CAD build for the part. Positions are in the model's coordinates, mm. A direction names the side the tool comes from. Coordinates: 2 decimals unless noted, no trailing zeros. Loops run counter-clockwise (first coordinate to the right, second up) from the corner with the lowest first, then second, coordinate; pieces in that order, holes last. Notation, with made-up numbers: (-28, 0.5) -> (26, 0.5) arc R6 cw to (26, 8.5) -> close; hole circle Ø3 at (57, -3.5). An arc over 180 degrees is marked (long way). Write each question's results on one line, items separated by ' | '.
Autodesk Inventor part; units mm, degrees
ref_plane "Work Plane1" through (0, -2.54, 0) normal (0, -1, 0) x (1, 0, 0)
ref_plane "YZ Plane" through (0, 0, 0) normal (1, 0, 0) x (0, 1, 0)
ref_plane "XZ Plane" through (0, 0, 0) normal (0, 1, 0) x (-1, 0, 0)
sketch "Sketch1" plane through (0, 0, 0) normal (0, 1, 0) x (-1, 0, 0)
  arc A0 (8.89, 11.1125) -> (-8.89, 11.1125) centre (0, 11.1125) ccw
  line L0 (-8.89, 0) -> (8.89, 0)
  arc A1 (-8.89, -11.1125) -> (8.89, -11.1125) centre (0, -11.1125) ccw
  line L1 (8.89, 11.1125) -> (8.89, -11.1125)
  line L2 (-8.89, 11.1125) -> (-8.89, -11.1125)
  point P0 (0, 0)
extrude "Extrusion1" add sketch "Sketch1" along normal blind 5.588
sketch "Sketch2" plane through (0, 5.588, 0) normal (0, 1, 0) x (1, 0, 0)
  arc A0 (-7.62, -11.1125) -> (7.62, -11.1125) centre (0, -11.1125) ccw
  arc A1 (7.62, 11.1125) -> (-7.62, 11.1125) centre (0, 11.1125) ccw
  line L0 (-7.62, -11.1125) -> (-7.62, 11.1125)
  line L1 (7.62, -11.1125) -> (7.62, 11.1125)
  line L2 (8.89, -11.1125) -> (8.89, 11.1125)
  line L3 (-8.89, 11.1125) -> (-8.89, -11.1125)
  arc A2 (-8.89, -11.1125) -> (8.89, -11.1125) centre (0, -11.1125) ccw
  point P0 (0, 0)
  dimension "d32" = 1.27
  dimension "d33" = 1.27
  dimension "d34" = 1.27
  dimension "d36" = 22.225
  dimension "d37" = 22.225
  dimension "d38" = 22.225
extrude "Extrusion2" cut sketch "Sketch2" against normal blind 0.508
sketch "Sketch3" plane through (0, 5.08, 0) normal (0, 1, 0) x (1, 0, 0)
  circle A0 centre (0, 0) radius 3.175
  point P0 (0, 0)
  dimension "d10" = 6.35
hole "Hole1" at (0, 5.08, 0) direction (0, -1, 0) diameter 6.35 end through all
thread "Thread1"
sketch "Sketch4" plane through (8.89, 0, 11.1125) normal (1, 0, 0) x (0, 0, -1)
  line L0 (5.0165, 0) -> (-12.6241, 2.794)
  line L1 (-12.6241, 2.794) -> (-8.89, 2.2026)
  line L2 (-8.89, 0) -> (-8.89, 5.588)
  line L3 (-8.89, 2.2026) -> (-8.89, 0)
  line L4 (5.0165, 0) -> (-8.89, 0)
  line L5 (-8.89, 2.2026) -> (5.0165, 0)
  point P0 (11.1125, 0)
  dimension "d29" = 9
  dimension "d30" = 6.096
extrude "Extrusion3" cut sketch "Sketch4" against normal through all
ref_plane "Work Plane1" through (0, -2.54, 0) normal (0, -1, 0) x (1, 0, 0)
sketch "Sketch5" plane through (0, -2.54, 0) normal (0, -1, 0) x (1, 0, 0)
  circle A0 centre (0, 13.716) radius 6.35
  line L0 (-5.5625, 10.6531) -> (5.5625, 16.7789)
  point P0 (0, 0)
  dimension "d23" = 12.7
  dimension "d31" = 13.716
revolve "Revolution1" cut sketch "Sketch5" angle 360 about axis through (-5.5625, -2.54, 10.6531) along (0.8759844, 0, 0.4823395) picked at (2.4961, 12.478) contours A0 L0
sketch "Sketch6" plane through (0, 0, 0) normal (0, -1, 0) x (1, 0, 0)
  circle A0 centre (0, -11.1125) radius 2.286
  point P0 (0, 0)
  dimension "d25" = 4.572
  dimension "d26" = 11.1125
extrude "Extrusion4" add sketch "Sketch6" along normal blind 1.27
properties part number "Lopez_LeftClamp" material "Polypropylene"
1) Which spindle directions (+Z, -Z, +X, -X, +Y, -Y) get a long thin tool onto all of the face, cutting with end or side? Do faces 5 (the cylindrical face through (-0.17, 5.34, 18.73)), 6 (the cylindrical face through (-0.5, -0.63, -8.88)), 7 (the cylindrical face through (3.1, 2.5, -0.69)). Say none if no direction does.
Outcome:
face 5: +Y | face 6: -Y | face 7: +Y, -Y
2) Pin check, flat tips, straight feed: pin 1 (3 mm diameter, centred on x = 5, z = -2.5, fed in from -Y); pin 2 (8.5 mm diameter, centred on x = 0, z = 0, fed in from +Y); pin 3 (4 mm diameter, centred on x = 1, y = 4.5, fed in from -Z); pin 4 (4 mm diameter, centred on y = 3, z = 14, fed in from -X). Stop position of each tip, or through.
Outcome:
pin 1: stops at y = 0 | pin 2: stops at y = 5.08 | pin 3: stops at z = -20 | pin 4: stops at x = -8.85
3) Slice it at A-A (z = 0). Write the cut outline in (x, y) (3 decimals), then the cut area to 3 significant figures.
Outcome:
outline: (-8.89, 0) -> (-3.175, 0) -> (-3.175, 5.08) -> (-7.62, 5.08) -> (-7.62, 5.588) -> (-8.89, 5.588) -> close; (3.175, 0) -> (8.89, 0) -> (8.89, 5.588) -> (7.62, 5.588) -> (7.62, 5.08) -> (3.175, 5.08) -> close | area: 59.4 mm^2
4) Drill centre lines: L1, parallel to X at y = 1.3, z = 0 (3 decimals); L2, parallel to Z at x = 0, y = 2.7 (1 decimal); L3, parallel to Z at x = -2, y = 2.5. Where is each one in solid material? Low to high. Write a range as from..to.
Outcome:
L1: x = -8.89..-3.175, 3.175..8.89 | L2: z = -20..-3.2, 3.2..10.1, 17.3..20 | L3: z = -19.77..-2.47, 2.47..10.41, 17.02..19.77
5) Two-plate mould, pull along X, no slides. Class faces 1 (the flat face through (0, -1.27, -11)), 2 (the flat face through (-3.5, 5.08, -0.3)), 3 (the cylindrical face through (0.2, 3.7, 20)), 4 (the flat face through (8.89, 3, 0)): pulls with the +X half, pulls with the -X half, needs draft (parallel to the pull), parting line crosses it, or undercut.
Outcome:
face 1: needs draft | face 2: undercut | face 3: parting line crosses it | face 4: pulls with the +X half
6) Slice it at D-D (z = 17). Write the cut outline in (x, y).
Outcome:
outline: (-6.66, 1.73) -> (-3.37, 1.73) arc R5.43 cw to (3.37, 1.73) -> (6.66, 1.73) -> (6.66, 5.59) -> (4.84, 5.59) -> (4.84, 5.08) -> (-4.84, 5.08) -> (-4.84, 5.59) -> (-6.66, 5.59) -> close
7) Slice it at C-C (y = 3). Count the separate pieces of the cut face and the enclosed holes in it, then the cut area to 3 significant figures.
Outcome:
separate pieces: 1 | enclosed holes: 2 | area: 582 mm^2
